```python
from build123d import *

# Parameters (mm, degrees)
SKETCH_1_R             = 7
EXTRUDE_1_DEPTH        = 160
EXTRUDE_1_DEPTH_BACK   = 36
SKETCH_2_R             = 7
EXTRUDE_2_DEPTH        = 8
SKETCH_3_W             = 18
SKETCH_3_H             = 11
EXTRUDE_3_DEPTH        = 15
EXTRUDE_4_DEPTH        = 30
SKETCH_5_W             = 60
SKETCH_5_H             = 40
EXTRUDE_5_DEPTH        = 6
SKETCH_6_W             = 60
SKETCH_6_H             = 6
EXTRUDE_6_DEPTH        = 60
SKETCH_7_W             = 29.455878384
SKETCH_7_H             = 4
EXTRUDE_7_DEPTH        = 8
PATTERN_LINEAR_1_COUNT = 2
PATTERN_LINEAR_1_PITCH = 52
SKETCH_8_W             = 71.56654599
SKETCH_8_H             = 41.958718016
CUT_EXTRUDE_1_DEPTH    = 300


with BuildPart() as part:
    # 草图1 → 凸台-拉伸1 (new body, two sides)
    with BuildSketch(Plane.XY) as extrude_1_sk:
        Circle(SKETCH_1_R)
    extrude(amount=EXTRUDE_1_DEPTH)
    extrude(extrude_1_sk.sketch, amount=-EXTRUDE_1_DEPTH_BACK)

    # 草图2 → 凸台-拉伸2 (add)
    with BuildSketch(Plane(origin=(0, 0, -36), x_dir=(-1, 0, 0), z_dir=(0, 0, -1))):
        Polygon((20, 7.5), (15, 12.5), (-15, 12.5), (-20, 7.5), (-20, -7.5), (-15, -12.5), (15, -12.5), (20, -7.5), align=None)
        Circle(SKETCH_2_R, mode=Mode.SUBTRACT)
        Circle(SKETCH_2_R)
    extrude(amount=EXTRUDE_2_DEPTH)

    # 草图3 → 凸台-拉伸3 (add)
    with BuildSketch(Plane(origin=(0, 0, -44), x_dir=(-1, 0, 0), z_dir=(0, 0, -1))):
        Rectangle(SKETCH_3_W, SKETCH_3_H)
    extrude(amount=EXTRUDE_3_DEPTH)

    # 草图4 → 凸台-拉伸4 (add)
    with BuildSketch(Plane(origin=(0, 0, -59), x_dir=(-1, 0, 0), z_dir=(0, 0, -1))):
        with BuildLine():
            Line((-15, -12.5), (-15, 12.5))
            ThreePointArc((-15, 12.5), (-27.5, 0), (-15, -12.5))
        make_face()
        with BuildLine():
            ThreePointArc((-3.77502784, 5.5), (-8.385621722, 10.606601718), (-15, 12.5))
            Line((-15, 12.5), (-15, -12.5))
            ThreePointArc((-15, -12.5), (-8.385621722, -10.606601718), (-3.77502784, -5.5))
            Line((-3.77502784, -5.5), (-9, -5.5))
            Line((-9, -5.5), (-9, 5.5))
            Line((-9, 5.5), (-3.77502784, 5.5))
        make_face()
        with BuildLine():
            ThreePointArc((-2.5, 0), (-2.822928267, 2.822928267), (-3.77502784, 5.5))
            Line((-3.77502784, 5.5), (-9, 5.5))
            Line((-9, 5.5), (-9, -5.5))
            Line((-9, -5.5), (-3.77502784, -5.5))
            ThreePointArc((-3.77502784, -5.5), (-2.822928267, -2.822928267), (-2.5, 0))
        make_face()
        with BuildLine():
            ThreePointArc((3.77502784, -5.5), (2.5, 0), (3.77502784, 5.5))
            Line((3.77502784, 5.5), (-3.77502784, 5.5))
            ThreePointArc((-3.77502784, 5.5), (-2.822928267, 2.822928267), (-2.5, 0))
            ThreePointArc((-2.5, 0), (-2.822928267, -2.822928267), (-3.77502784, -5.5))
            Line((-3.77502784, -5.5), (3.77502784, -5.5))
        make_face()
        with BuildLine():
            Line((9, 5.5), (3.77502784, 5.5))
            ThreePointArc((3.77502784, 5.5), (2.5, 0), (3.77502784, -5.5))
            Line((3.77502784, -5.5), (9, -5.5))
            Line((9, -5.5), (9, 5.5))
        make_face()
        with BuildLine():
            Line((15, -12.5), (15, 12.5))
            ThreePointArc((15, 12.5), (8.385621722, 10.606601718), (3.77502784, 5.5))
            Line((3.77502784, 5.5), (9, 5.5))
            Line((9, 5.5), (9, -5.5))
            Line((9, -5.5), (3.77502784, -5.5))
            ThreePointArc((3.77502784, -5.5), (8.385621722, -10.606601718), (15, -12.5))
        make_face()
        with BuildLine():
            ThreePointArc((27.5, 0), (23.838834765, 8.838834765), (15, 12.5))
            Line((15, 12.5), (15, -12.5))
            ThreePointArc((15, -12.5), (23.838834765, -8.838834765), (27.5, 0))
        make_face()
        with BuildLine():
            Line((-15, -12.5), (15, -12.5))
            ThreePointArc((15, -12.5), (8.385621722, -10.606601718), (3.77502784, -5.5))
            Line((3.77502784, -5.5), (-3.77502784, -5.5))
            ThreePointArc((-3.77502784, -5.5), (-8.385621722, -10.606601718), (-15, -12.5))
        make_face()
        with BuildLine():
            ThreePointArc((3.77502784, 5.5), (8.385621722, 10.606601718), (15, 12.5))
            Line((15, 12.5), (-15, 12.5))
            ThreePointArc((-15, 12.5), (-8.385621722, 10.606601718), (-3.77502784, 5.5))
            Line((-3.77502784, 5.5), (3.77502784, 5.5))
        make_face()
    extrude(amount=EXTRUDE_4_DEPTH)

    # 草图5 → 凸台-拉伸5 (add)
    with BuildSketch(Plane(origin=(0, 0, -89), x_dir=(-1, 0, 0), z_dir=(0, 0, -1))):
        Rectangle(SKETCH_5_W, SKETCH_5_H)
    extrude(amount=EXTRUDE_5_DEPTH)

    # 草图6 → 凸台-拉伸6 (add)
    with BuildSketch(Plane(origin=(0, 0, -95), x_dir=(-1, 0, 0), z_dir=(0, 0, -1))):
        with Locations((0, 17)):
            Rectangle(SKETCH_6_W, SKETCH_6_H)
        with Locations((0, -17)):
            Rectangle(SKETCH_6_W, SKETCH_6_H)
    extrude(amount=EXTRUDE_6_DEPTH)

    # 草图7 → 凸台-拉伸7 (add)
    with BuildSketch(Plane.ZY.offset(30)):
        Polygon((-125, 8), (-125, 14), (-155, 14), (-160, 14), (-160, 8), align=None)
        Polygon((-125, -8), (-160, -8), (-160, -14), (-155, -14), (-125, -14), align=None)
        Polygon((-160, 8), (-160, 14), (-166, 14), (-166, 4), (-166, 0), (-166, -4), (-166, -14), (-160, -14), (-160, -8), align=None)
        with Locations((-180.727939192, -2)):
            Rectangle(SKETCH_7_W, SKETCH_7_H)
        with Locations((-180.727939192, 2)):
            Rectangle(SKETCH_7_W, SKETCH_7_H)
    extrude_7 = extrude(amount=-EXTRUDE_7_DEPTH)

    # 阵列(线性)1: 凸台-拉伸7 ×2
    with Locations(*[(i * PATTERN_LINEAR_1_PITCH, 0, 0) for i in range(1, PATTERN_LINEAR_1_COUNT)]):
        add(extrude_7)

    # 草图8 → 切除-拉伸1 (cut)
    with BuildSketch(Plane.XY.offset(-59)):
        Rectangle(SKETCH_8_W, SKETCH_8_H)
    extrude(amount=CUT_EXTRUDE_1_DEPTH, mode=Mode.SUBTRACT)


solid = part.part
```
Input: part model. Units: mm. Frame: model coordinates. A direction names the side the tool comes from. Round coordinates to 2 decimals unless told otherwise and drop trailing zeros. Write each loop counter-clockwise with the first axis right and the second up, starting at its lowest first coordinate (ties: lowest second). Pieces come first, ordered by that corner, then holes. Notation, with made-up numbers: (70.25, 19) - (118.25, 19) arc R24 ccw to (118.25, 40) - close; hole circle Ø7 at (36, -26). An arc over 180 degrees is marked (long way). Write item = value, one per line.
(1) Section query D-D on z = -68. Output: boundary loops of the cut face in (x, y).
Geometry check:
outline = (-15, -12.5) - (15, -12.5) arc R12.5 ccw to (15, 12.5) - (-15, 12.5) arc R12.5 ccw to start
(2) Section query C-C on z = -100.5. Output: boundary loops of the cut face in (x, y), then the cut area to 3 significant figures.
Geometry check:
outline = (-30, -20) - (30, -20) - (30, -14) - (-30, -14) - close; (-30, 14) - (30, 14) - (30, 20) - (-30, 20) - close
area = 720 mm^2
(3) Material intervals for probe 1 along Z at (x, y) = (25.5, -7); probe 2 along Y at (x, z) = (-25, -97); probe 3 along Z at (x, y) = (27, -11), sorted ascending.
Geometry check:
probe_1 = -166 to -160, -95 to -89
probe_2 = -20 to -14, 14 to 20
probe_3 = -166 to -125, -95 to -89
(4) Section query A-A on z = -169. Output: boundary loops of the cut face in (x, y), then the cut area to 3 significant figures.
Geometry check:
outline = (-30, -4) - (-22, -4) - (-22, 4) - (-30, 4) - close; (22, -4) - (30, -4) - (30, 4) - (22, 4) - close
area = 128 mm^2
(5) Pull-direction query (Y, two-part tool) for faces 1 (the flat face through (30, -10, -135)), 2 (the flat face through (26, 8, -143)), 3 (the flat face through (26, 14, -160)), 4 (the cylindrical face through (27.497, 0.275, -73.79)); classes: +Y half, -Y half, draft (parallel to the pull), parting line (faces both ways), or undercut.
Geometry check:
face_1 = draft
face_2 = undercut
face_3 = +Y half
face_4 = parting line
(6) Contact query for flat-ended pins moving along their axis: pin 1 Ø6.5 at (x, z) = (-24.5, -174.5) entering from +Y; pin 2 Ø2.5 at (x, y) = (-25, -11) entering from -Z; pin 3 Ø12 at (x, z) = (14, -73) entering from +Y. Output: stop coordinate, or through.
Geometry check:
pin_1 = 4
pin_2 = -166
pin_3 = 12.5
(7) Section query B-B on x = -23.5. Output: boundary loops of the cut face in (y, z), then the cut area to 3 significant figures.
Geometry check:
outline = (-20, -155) - (-14, -155) - (-14, -166) - (-4, -166) - (-4, -195.46) - (4, -195.46) - (4, -166) - (14, -166) - (14, -155) - (20, -155) - (20, -89) - (9.17, -89) - (9.17, -59) - (-9.17, -59) - (-9.17, -89) - (-20, -89) - close; hole (-14, -125) - (-8, -125) - (-8, -160) - (8, -160) - (8, -125) - (14, -125) - (14, -95) - (-14, -95) - close
area = 2,330 mm^2
(8) Access query for faces 5 (the flat face through (-22, 0, -161)), 6 (the flat face through (-26, 9, -166)), 7 (the flat face through (26, -8, -142)), 8 (the flat face through (0, 12.5, -74)), 9 (the flat face through (26, -9, -166)). Directions: +Z, -Z, +X, -X, +Y, -Y. A direction counts if a zero-diameter tool reaches every point of the face in a straight line with its end or side. Return the directions, or none.
Geometry check:
face_5 = -Z
face_6 = -Z, +X, -X, +Y
face_7 = +X, -X
face_8 = +Z, +X, -X, +Y
face_9 = -Z, +X, -X, -Y
